from build123d import *

# Parameters (mm, degrees)
F1_DEPTH = 2.54
F3_DEPTH = 25.4
F5_DEPTH = 2.032
F7_DEPTH = 1.27
F8_SIZE  = 1.27


with BuildPart() as f1:
    # F0 (on Front) → F1 (new body)
    with BuildSketch(Plane.XZ):
        with BuildLine():
            ThreePointArc((33.00001, 49.374628), (16.500005, 51.000006), (0, 49.374628))
            Line((0, 49.374628), (0, 0))
            Line((0, 0), (33.00001, 0))
            Line((33.00001, 0), (33.00001, 49.374628))
        make_face()
    extrude(amount=F1_DEPTH)

    # F2 (on face) → F3 (cut)
    with BuildSketch(Plane.XZ.offset(2.54)):
        Polygon((20.581914, 25.74524), (16.500005, 32.815314), (12.418096, 25.74524), (13.737919, 24.98324), (16.500005, 29.767314), (19.262091, 24.98324), align=None)
        Polygon((11.783096, 24.645388), (7.701187, 17.575314), (15.865005, 17.575314), (15.865005, 19.099314), (10.340832, 19.099314), (13.102919, 23.883388), align=None)
        Polygon((17.135005, 17.575314), (25.298823, 17.575314), (21.216914, 24.645388), (19.897091, 23.883388), (22.659178, 19.099314), (17.135005, 19.099314), align=None)
        Polygon((32.22455, 13.589), (26.358671, 13.589), (27.3852, 11.811), (27.971787, 11.811), (27.238553, 13.081), (29.29161, 13.081), (31.344668, 13.081), (30.611433, 11.811), (31.198021, 11.811), align=None)
        Polygon((27.678494, 11.303), (29.29161, 8.509), (30.904727, 11.303), (30.318139, 11.303), (29.29161, 9.525), (28.265081, 11.303), align=None)
        Polygon((1.801989, 38.071628), (0.775461, 36.293628), (6.641339, 36.293628), (5.614811, 38.071628), (5.028223, 38.071628), (5.761458, 36.801628), (1.655342, 36.801628), (2.388577, 38.071628), align=None)
        Polygon((5.321517, 38.579628), (3.7084, 41.373628), (2.095283, 38.579628), (2.681871, 38.579628), (3.7084, 40.357628), (4.734929, 38.579628), align=None)
    extrude(amount=-F3_DEPTH, mode=Mode.SUBTRACT)

    # F4 (on face) → F5 (cut)
    with BuildSketch(Plane.XZ.offset(2.54)):
        Polygon((6.641339, 36.293628), (3.7084, 41.373628), (0.775461, 36.293628), align=None)
        Polygon((1.655342, 36.801628), (3.7084, 40.357628), (5.761458, 36.801628), align=None, mode=Mode.SUBTRACT)
        Polygon((32.22455, 13.589), (26.358671, 13.589), (29.29161, 8.509), align=None)
        Polygon((29.29161, 9.525), (27.238553, 13.081), (31.344668, 13.081), align=None, mode=Mode.SUBTRACT)
    extrude(amount=-F5_DEPTH, mode=Mode.SUBTRACT)

    # F6 (on face) → F7 (cut)
    with BuildSketch(Plane.XZ.offset(2.54)):
        Polygon((25.298823, 17.575314), (16.500005, 32.815314), (7.701187, 17.575314), align=None)
        Polygon((10.340832, 19.099314), (16.500005, 29.767314), (22.659178, 19.099314), align=None, mode=Mode.SUBTRACT)
    extrude(amount=-F7_DEPTH, mode=Mode.SUBTRACT)

    # F8
    f8_edges = [f1.edges().sort_by_distance(p)[0] for p in [
        (23.257869, 0, 21.110351),
        (18.54096, 0, 29.280277),
        (9.742142, 0, 21.110351),
        (14.459051, 0, 29.280277),
        (11.783096, 0, 17.575314),
        (21.216914, 0, 17.575314),
        (21.278135, 0, 21.491351),
        (17.881048, 0, 27.375277),
        (13.102919, 0, 19.099314),
        (19.897091, 0, 19.099314),
        (11.721876, 0, 21.491351),
        (15.118962, 0, 27.375277),
    ]]
    chamfer(f8_edges, length=F8_SIZE)


solid = f1.part
Work out the finished part from the listing and answer in its coordinate system (mm). A direction names the side the tool comes from. Round coordinates to 2 decimals unless told otherwise and drop trailing zeros. Write each loop counter-clockwise with the first axis right and the second up, starting at its lowest first coordinate (ties: lowest second). Pieces come first, ordered by that corner, then holes. Notation, with made-up numbers: (29.5, 63.25) -> (52.5, 63.25) arc R21 ccw to (52.5, 102.25) -> close; hole circle Ø11 at (-27.75, -3.75). An arc over 180 degrees is marked (long way). Answer as CSV lines item,"result". Start each with the question number.
(1) The mould has two halves that part along Z. Classify faces 4 (the flat face through (33, -1, 24)), 5 (the flat face through (4, -1, 36.294)): +Z half, -Z half, draft (parallel to the pull), parting line (faces both ways), or undercut.
(2) Find the intervals of material crossed by probe 1 along X at (y, z) = (-0.85, 24); probe 2 along X at (y, z) = (-0.5, 19.5) (3 decimals); probe 3 along Z at (x, y) = (2, -2.25), in increasing order.
(3) The part is cut by section A-A, the plane y = -2.15. Give the vertices of the cut face in (x, z) (3 decimals).
(4) The part is cut by section D-D, the plane z = 17. Give the vertices of the cut face in (x, y) (3 decimals).
(5) Each of these flat-tipped pins is pushed along its axis until it touches: pin 1 (0.6 mm diameter, centred on x = 28, y = -0.5, fed in from -Z); pin 2 (1.5 mm diameter, centred on x = 14.5, y = -0.5, fed in from +Z); pin 3 (0.6 mm diameter, centred on x = 5, y = -0.5, fed in from +Z) (3 decimals); pin 4 (0.6 mm diameter, centred on x = 2.5, y = -0.5, fed in from +Z). Where does it stop, or does it pass through?
(6) The part is cut by section B-B, the plane z = 39.5. Give the vertices of the cut face in (x, y).
(7) A tool of negligible diameter and unlimited length cuts with its end or side. For faces 1 (the flat face through (15.1, -1.91, 27.34)), 2 (the flat face through (19.32, -0.63, 19.74)), 3 (the flat face through (20, -2.54, 32)), from which of +Z, -Z, +X, -X, +Y, -Y can it reach the whole face along a straight path? Write none if from no direction.
(8) The part is cut by section C-C, the plane x = 24. Give the vertices of the cut face in (y, z), then the cut area to 3 significant figures.
Output values:
1,face 4,"draft"
1,face 5,"undercut"
2,probe 1,"x = 0 to 10.93, 12.9 to 20.1, 22.07 to 33"
2,probe 2,"x = 0 to 7.923, 15.865 to 17.135, 25.077 to 33"
2,probe 3,"z = 0 to 36.29, 36.8 to 37.4, 38.41 to 49.75"
3,outline,"(0, 0) -> (33, 0) -> (33, 49.375) arc R84.562 ccw to (0, 49.375) -> close; (1.655, 36.802) -> (5.761, 36.802) -> (3.708, 40.358) -> close; (10.341, 19.099) -> (22.659, 19.099) -> (16.5, 29.767) -> close; (27.239, 13.081) -> (29.292, 9.525) -> (31.345, 13.081) -> close; hole (0.775, 36.294) -> (6.641, 36.294) -> (5.615, 38.072) -> (5.322, 38.58) -> (3.708, 41.374) -> (2.095, 38.58) -> (1.802, 38.072) -> close; hole (7.701, 17.575) -> (25.299, 17.575) -> (16.5, 32.815) -> close; hole (26.359, 13.589) -> (29.292, 8.509) -> (32.225, 13.589) -> close"
4,outline,"(0, -2.54) -> (33, -2.54) -> (33, 0) -> (27.097, 0) -> (26.295, -0.695) -> (17.135, -0.695) -> (17.135, 0) -> (15.865, 0) -> (15.865, -0.695) -> (6.705, -0.695) -> (5.903, 0) -> (0, 0) -> close"
5,pin 1,"stops at z = 0"
5,pin 2,"stops at z = 50.99"
5,pin 3,"stops at z = 50.255"
5,pin 4,"stops at z = 49.88"
6,outline,"(0, -2.54) -> (2.63, -2.54) -> (2.63, 0) -> (0, 0) -> close; (3.21, -2.54) -> (4.2, -2.54) -> (4.2, 0) -> (3.21, 0) -> close; (4.79, -2.54) -> (33, -2.54) -> (33, 0) -> (4.79, 0) -> close"
7,face 1,"+Y, -Y"
7,face 2,"+Y"
7,face 3,"+Z, -Z, +X, -X, -Y"
8,outline,"(-2.54, 0) -> (0, 0) -> (0, 16.31) -> (-1.27, 17.58) -> (-2.54, 17.58) -> close; (-2.54, 19.82) -> (-1.27, 19.82) -> (0, 22.36) -> (0, 50.67) -> (-2.54, 50.67) -> close"
8,area,"121 mm²"
